Input: dimensioned drawing with shaded views. Units: mm. Origin: part minimum x, y, z. Give positions to 0.01 mm unless a question says otherwise; leave off trailing zeros. Write each loop counter-clockwise with the first axis right and the second up, starting at its lowest first coordinate (ties: lowest second). Pieces come first, ordered by that corner, then holes. Notation, with made-up numbers: (1.25, 1) -> (59.25, 1) arc R25 ccw to (59.25, 23) -> close; hole circle Ø11 at (41, -19). An arc over 180 degrees is marked (long way). Answer as a JSON object with one key per item and string values.
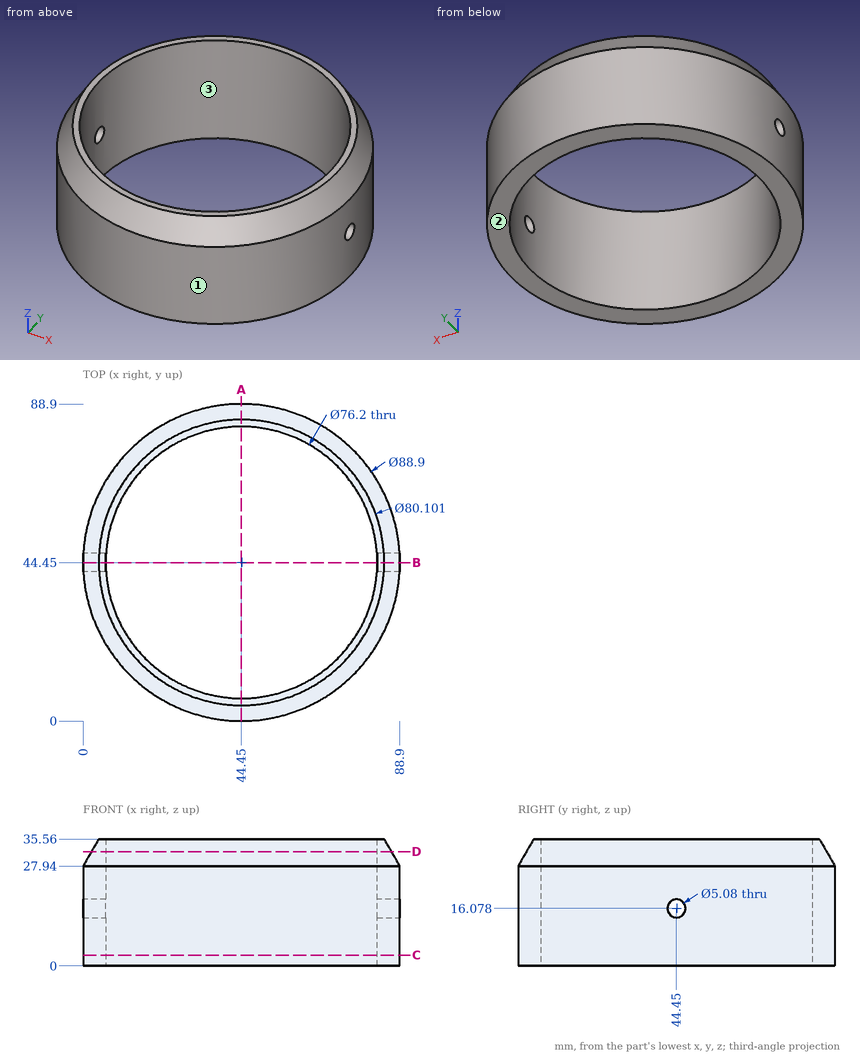
Q1. Cut plane B-B (y = 44.45). Return the cut outline in (x, z).
Values:
{"outline": "(0, 0) -> (6.35, 0) -> (6.35, 13.54) -> (0, 13.54) -> close; (0, 18.62) -> (6.35, 18.62) -> (6.35, 35.56) -> (4.4, 35.56) -> (0, 27.94) -> close; (82.55, 0) -> (88.9, 0) -> (88.9, 13.54) -> (82.55, 13.54) -> close; (82.55, 18.62) -> (88.9, 18.62) -> (88.9, 27.94) -> (84.5, 35.56) -> (82.55, 35.56) -> close"}
Q2. Cut plane A-A (x = 44.45). Return the cut outline in (y, z).
Values:
{"outline": "(0, 0) -> (6.35, 0) -> (6.35, 35.56) -> (4.4, 35.56) -> (0, 27.94) -> close; (82.55, 0) -> (88.9, 0) -> (88.9, 27.94) -> (84.5, 35.56) -> (82.55, 35.56) -> close"}
Q3. First-contact query: P1, Ø12, axis at x = 20.5, z = 19.5, coming from the +Y side; P2, Ø6, axis at y = 66.5, z = 23, coming from the +X side; P3, Ø12, axis at x = 50, z = 18.5, coming from the +Y side. Flat tips, straight axial feed; report the tip coordinate or a pass-through.
Values:
{"P1": "y = 85.11", "P2": "x = 84.61", "P3": "y = 88.9"}
Q4. Material intervals for L1, parallel to Y at x = 44, z = 26; L2, parallel to Z at x = 85, y = 44, sorted ascending. Write a range as from..to.
Values:
{"L1": "0..6.35, 82.55..88.9", "L2": "0..13.58, 18.58..34.69"}
Q5. Cut plane C-C (z = 3). Return the cut outline in (x, y), and give its area (3 significant figures).
Values:
{"outline": "circle Ø88.9 at (44.45, 44.45); hole circle Ø76.2 at (44.45, 44.45)", "area": "1,650 mm²"}
Q6. Cut plane D-D (z = 32). Return the cut outline in (x, y).
Values:
{"outline": "circle Ø84.21 at (44.45, 44.45); hole circle Ø76.2 at (44.45, 44.45)"}
Q7. Mould query, pull axis X, two halves, no side actions, for the marked faces 1, 2 and 3. Classes: pulls with the +X half, pulls with the -X half, needs draft (parallel to the pull), parting line crosses it, or undercut.
Values:
{"face 1": "parting line crosses it", "face 2": "needs draft", "face 3": "undercut"}
